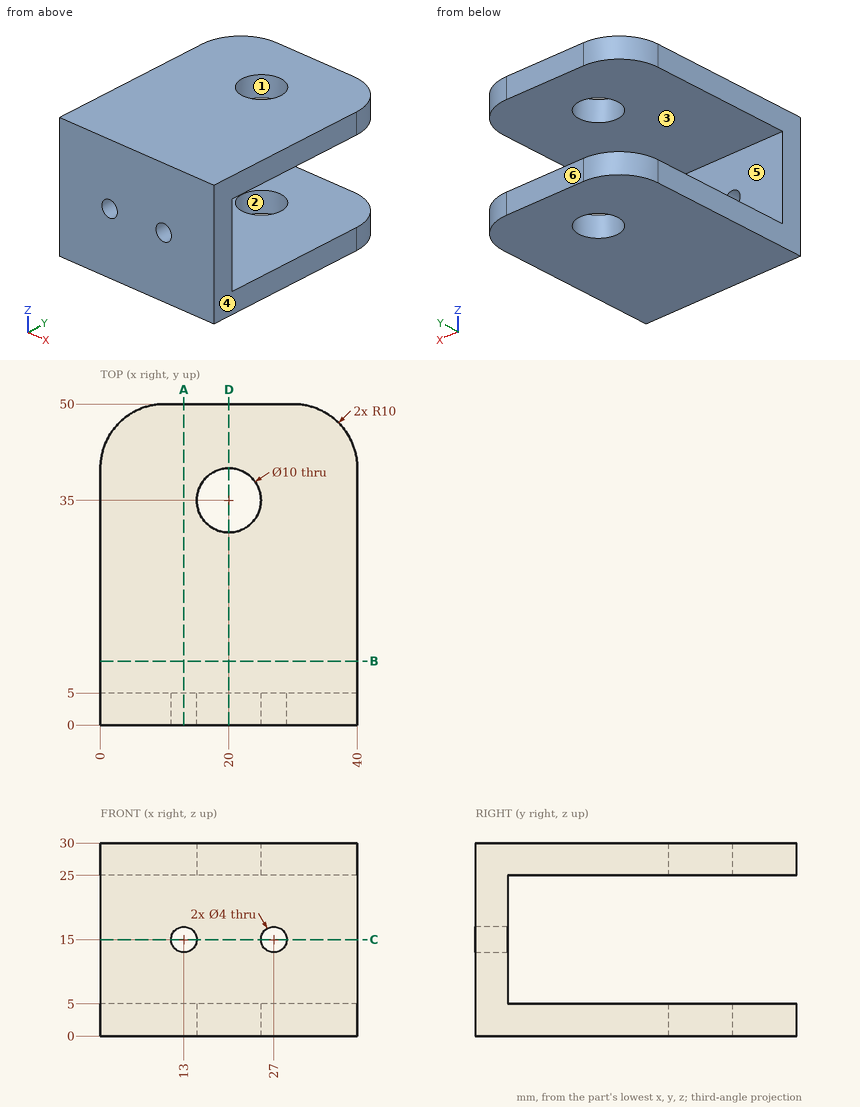
Here's the drawing with two shaded views (mm, measured from the low corner). I have some questions. A direction names the side the tool comes from. Round coordinates to 2 decimals unless told otherwise and drop trailing zeros. Write each loop counter-clockwise with the first axis right and the second up, starting at its lowest first coordinate (ties: lowest second). Pieces come first, ordered by that corner, then holes. Notation, with made-up numbers: M -37,11 L 8,11 A12 cw 8,16 Z; hole C -10.5,48 d3. An arc over 180 degrees is marked long. Use CSV: the item, a comma, the result in double quotes.
(1) Imagine slicing it at A-A (x = 13). Write out the boundary of the cut face in (y, z), plus the area to 3 significant figures.
Check values:
outline,"M 0,0 L 50,0 L 50,5 L 5,5 L 5,13 L 0,13 Z; M 0,17 L 5,17 L 5,25 L 50,25 L 50,30 L 0,30 Z"
area,"580 mm^2"
(2) On a 3-axis mill with a long thin cutter (end or side, diameter ignored), from which of +Z, -Z, +X, -X, +Y, -Y can I reach the whole of each face in a straight line? I mean the marked faces 5 and 6. Say none if no direction works.
Check values:
face 5,"+X, -X, +Y"
face 6,"+Z, -Z, +X, -X, +Y"
(3) We'd pull the mould along X, two halves only. Please class the marked faces 1, 2, 3 and 4: +X half, -X half, draft (parallel to the pull), parting line (faces both ways), or undercut.
Check values:
face 1,"undercut"
face 2,"undercut"
face 3,"draft"
face 4,"+X half"
(4) Imagine slicing it at D-D (x = 20). Write out the boundary of the cut face in (y, z), plus the area to 3 significant figures.
Check values:
outline,"M 0,0 L 30,0 L 30,5 L 5,5 L 5,25 L 30,25 L 30,30 L 0,30 Z; M 40,0 L 50,0 L 50,5 L 40,5 Z; M 40,25 L 50,25 L 50,30 L 40,30 Z"
area,"500 mm^2"
(5) Imagine slicing it at B-B (y = 10). Write out the boundary of the cut face in (x, z), plus the area to 3 significant figures.
Check values:
outline,"M 0,0 L 40,0 L 40,5 L 0,5 Z; M 0,25 L 40,25 L 40,30 L 0,30 Z"
area,"400 mm^2"
(6) I'm going to push flat-ended pins straight in: pin 1 (9 mm diameter, centred on x = 20, y = 35, fed in from +Z); pin 2 (5 mm diameter, centred on x = 27, z = 15, fed in from +Y). Where does each tip first touch, or does it pass through?
Check values:
pin 1,"through"
pin 2,"y = 5"
(7) I need wall thicknesses on line 1 along X through (y, z) = (2.85, 15); line 2 along Z through (x, y) = (25, 22); line 3 along X through (y, z) = (35, 3.95). Which ranges of each line are inside material? Lowest first, please.
Check values:
line 1,"0 to 11, 15 to 25, 29 to 40"
line 2,"0 to 5, 25 to 30"
line 3,"0 to 15, 25 to 40"
(8) Imagine slicing it at C-C (z = 15). Write out the boundary of the cut face in (x, y), plus the area to 3 significant figures.
Check values:
outline,"M 0,0 L 11,0 L 11,5 L 0,5 Z; M 15,0 L 25,0 L 25,5 L 15,5 Z; M 29,0 L 40,0 L 40,5 L 29,5 Z"
area,"160 mm^2"
